Autodesk Inventor part; units mm, degrees
ref_plane "YZ Plane" through (0, 0, 0) normal (1, 0, 0) x (0, 1, 0)
ref_plane "XZ Plane" through (0, 0, 0) normal (0, 1, 0) x (-1, 0, 0)
ref_plane "XY Plane" through (0, 0, 0) normal (0, 0, 1) x (1, 0, 0)
sketch "Sketch1" plane through (0, 0, 0) normal (0, 1, 0) x (-1, 0, 0)
  circle A0 centre (0, 0) radius 90
  line L0 (73.4575, 52) -> (-73.4575, 52)
  dimension "d0" = 180
  dimension "d1" = 52
extrude "Extrusion1" add sketch "Sketch1" along normal blind 3 contours A0 L0 picked at (17.1608, -0.9679)
sketch "Sketch2" plane through (0, 3, 0) normal (0, 1, 0) x (1, 0, 0)
  line L0 (-73.4575, -52) -> (73.4575, -52)
  line L1 (60, -52) -> (-90, -52)
  line L2 (-90, -52) -> (-90, 90)
  line L3 (-90, 90) -> (60, 90)
  line L4 (60, 90) -> (60, -52)
  arc A0 (73.4575, -52) -> (-73.4575, -52) centre (0, 0) ccw
  dimension "d4" = 60
extrude "Extrusion2" cut sketch "Sketch2" against normal blind 3 contours A0 L4 L0 | L1 L2 A0 | L2 L3 A0 | A0 L3 L4 picked at (-22.3183, 24.985)
sketch "Sketch3" plane through (0, 3, 0) normal (0, 1, 0) x (1, 0, 0)
  line L0 (60, 67.082) -> (45, 67.082)
  line L1 (45, 67.082) -> (45, 43)
  line L2 (45, 43) -> (60, 43)
  line L3 (60, 43) -> (60, 67.082)
  line L4 (60, -52) -> (73.4575, -52)
  line L5 (60, -52) -> (57, -52)
  line L6 (57, -52) -> (57, -47)
  line L7 (57, -47) -> (60, -47)
  line L8 (60, -47) -> (60, -52)
  point P0 (0, 0)
  dimension "d7" = 15
  dimension "d8" = 95
  dimension "d9" = 3
  dimension "d10" = 5
extrude "Extrusion3" add sketch "Sketch3" against normal blind 3
sketch "Sketch4" plane through (0, 3, 0) normal (0, 1, 0) x (1, 0, 0)
  line L0 (60, -47) -> (60, 43)
  line L1 (60, -45) -> (70, -45)
  line L2 (70, -45) -> (70, 15)
  line L3 (70, 15) -> (60, 15)
  line L4 (60, 15) -> (60, -45)
  line L5 (57, -52) -> (73.4575, -52)
  point P0 (0, 0)
  dimension "d13" = 10
  dimension "d14" = 60
  dimension "d15" = 7
extrude "Extrusion4" cut sketch "Sketch4" against normal blind 3
sketch "Sketch5" plane through (0, 3, 0) normal (0, 1, 0) x (1, 0, 0)
  line L0 (75, -1.5) -> (85, -1.5)
  line L1 (85, -1.5) -> (85, 1.5)
  line L2 (85, 1.5) -> (75, 1.5)
  line L3 (75, 1.5) -> (75, -1.5)
  line L4 (70, -45) -> (70, 15)
  point P0 (0, 0)
  point P1 (75, 0)
  dimension "d18" = 10
  dimension "d19" = 3
  dimension "d20" = 5
extrude "Extrusion5" cut sketch "Sketch5" against normal blind 3
sketch "Sketch6" plane through (0, 3, 0) normal (0, 1, 0) x (1, 0, 0)
  circle A0 centre (52, 48) radius 1.5
  circle A1 centre (52, 63) radius 1.5
  line L0 (60, 43) -> (60, 15)
  line L1 (45, 43) -> (60, 43)
  point P0 (0, 0)
  dimension "d23" = 3
  dimension "d24" = 3
  dimension "d25" = 15
  dimension "d26" = 8
  dimension "d27" = 5
extrude "Extrusion6" cut sketch "Sketch6" against normal blind 3
sketch "Sketch7" plane through (0, 3, 0) normal (0, 1, 0) x (1, 0, 0)
  line L0 (60, 43) -> (57, 43)
  line L1 (57, 43) -> (57, 38)
  line L2 (57, 38) -> (60, 38)
  line L3 (60, 38) -> (60, 43)
  point P0 (0, 0)
  dimension "d30" = 3
  dimension "d31" = 5
extrude "Extrusion7" add sketch "Sketch7" against normal blind 3
sketch "Sketch8" plane through (0, 3, 0) normal (0, 1, 0) x (1, 0, 0)
  line L0 (57, -52) -> (73.4575, -52)
  line L1 (62.5, -52) -> (67.5, -52)
  line L2 (67.5, -52) -> (67.5, -55)
  line L3 (67.5, -55) -> (62.5, -55)
  line L4 (62.5, -55) -> (62.5, -52)
  line L5 (60, -45) -> (60, -47)
  point P0 (0, 0)
  dimension "d34" = 5
  dimension "d35" = 3
  dimension "d36" = 2.5
extrude "Extrusion8" add sketch "Sketch8" against normal blind 3
properties part number "Out side rib"
CAD build for the part. Positions are in the model's coordinates, mm. A direction names the side the tool comes from. Round coordinates to 2 decimals unless told otherwise and drop trailing zeros. Order: outer loops, then holes, each group sorted by start corner. A loop starts at its lowest first (then second) coordinate and runs counter-clockwise, first axis right, second up. Notation, with made-up numbers: (-28.5, 6) - (25.5, 6) arc R22 ccw to (25.5, 16) - close; hole circle Ø5 at (-13.75, -25). An arc over 180 degrees is marked (long way). Use CSV: the item, a comma, the result in double quotes. Start each with the question number.
1) Saw through at D-D (x = 64.5). List the corners of the cut face in (y, z), and give its area (3 significant figures).
2) Pin check, flat tips, straight feed: pin 1 Ø1.5 at (y, z) = (1, 49) entering from -X; pin 2 Ø0.9 at (x, y) = (58, 1) entering from +Z; pin 3 Ø1.5 at (y, z) = (1, -31) entering from -X. Stop position of each tip, or through.
3) Saw through at A-A (x = 52). List the corners of the cut face in (y, z), and give its area (3 significant figures).
4) Saw through at C-C (y = 1.5). Count the separate pieces of the cut face and the enclosed holes in it, and give its area (3 significant figures).
5) Tool access for faces 5 (the flat face through (57, 2, -41)), 6 (the flat face through (85, 2, 0)), 7 (the flat face through (72, 3, -7)), 8 (the flat face through (65, 2, 45)): list every direction of +Z, -Z, +X, -X, +Y, -Y with a clear straight run to the whole face (end or side of a thin tool).
6) Wall check: L1, parallel to Z at x = 52, y = 0.75; L2, parallel to Z at x = 58, y = 1.6; L3, parallel to X at y = 1, z = -63. Give the ranges that are in metal, low to high. Write a range as [from, to].
7) Saw through at B-B (z = -48). List the corners of the cut face in (x, y).
8) Two-plate mould, pull along X, no slides. Class faces 1 (the flat face through (67.5, 2, 53)), 2 (the flat face through (75, 2, 0)), 3 (the flat face through (70, 2, 15)), 4 (the flat face through (70, 1, 52)): pulls with the +X half, pulls with the -X half, needs draft (parallel to the pull), parting line crosses it, or undercut.
Values follow:
1,outline,"(0, -62.77) - (3, -62.77) - (3, -15) - (0, -15) - close; (0, 45) - (3, 45) - (3, 55) - (0, 55) - close"
1,area,"173 mm2"
2,pin 1,"stops at x = 57"
2,pin 2,"stops at z = 52"
2,pin 3,"stops at x = 60"
3,outline,"(0, -67.08) - (3, -67.08) - (3, -64.5) - (0, -64.5) - close; (0, -61.5) - (3, -61.5) - (3, -49.5) - (0, -49.5) - close; (0, -46.5) - (3, -46.5) - (3, -43) - (0, -43) - close"
3,area,"54.2 mm2"
4,separate pieces,"1"
4,enclosed holes,"3"
4,area,"2,440 mm2"
5,face 5,"+Z, -X, +Y, -Y"
5,face 6,"+Y, -Y"
5,face 7,"+Z, -Z, +X, -X, +Y"
5,face 8,"-X, +Y, -Y"
6,L1,"z = [-67.08, -64.5], [-61.5, -49.5], [-46.5, -43]"
6,L2,"z = [-67.08, -38], [47, 52]"
6,L3,"x = [45, 50.5], [53.5, 64.27]"
7,outline,"(45, 0) - (50.5, 0) - (50.5, 3) - (45, 3) - close; (53.5, 0) - (76.13, 0) - (76.13, 3) - (53.5, 3) - close"
8,face 1,"pulls with the +X half"
8,face 2,"undercut"
8,face 3,"pulls with the -X half"
8,face 4,"needs draft"
